Source: CAD feature listing. Evaluate the final solid. Frame: model axes, mm. Face numbers are marked on the shaded views. A direction names the side the tool comes from. Coordinates: 2 decimals unless noted, no trailing zeros. Write each loop counter-clockwise with the first axis right and the second up, starting at its lowest first coordinate (ties: lowest second). Pieces come first, ordered by that corner, then holes. Notation, with made-up numbers: M 57,29.5 L 61,29.5 A27 cw 61,59.5 Z; hole C 21,19 d7. An arc over 180 degrees is marked long. Write item = value, one per line. Start each with the question number.
1. Line query: line 1 along Z through (x, y) = (1.3, 0) (3 decimals); line 2 along Y through (x, z) = (-2, -1.5); line 3 along Y through (x, z) = (3.4, 0) (3 decimals). Output: solid intervals per line, ascending.
2. Section query C-C (x = -2.5). Output: boundary loops of the cut face in (y, z).
3. Section query D-D (z = 3.25). Output: boundary loops of the cut face in (x, y), then the cut area to 3 significant figures.
4. Section query A-A (z = -1.75). Output: boundary loops of the cut face in (x, y).
5. Access query for the marked faces 1, 2 and 3. Directions: +Z, -Z, +X, -X, +Y, -Y. A direction counts if a zero-diameter tool reaches every point of the face in a straight line with its end or side. Return the directions, or none.
6. Section query B-B (y = 1.5). Output: boundary loops of the cut face in (x, z), then the cut area to 3 significant figures.
7. Pull-direction query (X, two-part tool) for the marked faces 4, 5 and 6; classes: pulls with the +X half, pulls with the -X half, needs draft (parallel to the pull), parting line crosses it, or undercut.
8. Pin query (flat end, axial travel): pin 1 Ø2.5 at (y, z) = (0, 0) entering from -X; pin 2 Ø1.1 at (x, y) = (-3.5, 1.5) entering from +Z. Return the tip coordinate at first contact, or that it passes through.
```python
from build123d import *

# Parameters (mm, degrees)
SKETCH052_W          = 12
SKETCH052_H          = 14
PAD011_DEPTH         = 6
POCKET024_DEPTH      = 1
POCKET025_DEPTH      = 5.001
SKETCH055_R          = 2.125
POCKET026_DEPTH      = 6.001
POCKET026_DEPTH_BACK = 6.001
SKETCH056_R          = 4.65
POCKET027_DEPTH      = 1


with BuildPart() as part:
    # Sketch052 → Pad011 (new body, symmetric)
    with BuildSketch(Plane.XY):
        Rectangle(SKETCH052_W, SKETCH052_H)
    extrude(amount=PAD011_DEPTH, both=True)

    # Sketch053 → Pocket024 (cut)
    with BuildSketch(Plane.YZ):
        with BuildLine():
            ThreePointArc((-4.65, 0), (0, -4.65), (4.65, 0))
            Line((4.65, 0), (4.65, 10))
            Line((4.65, 10), (-4.65, 10))
            Line((-4.65, 10), (-4.65, 0))
        make_face()
    extrude(amount=-POCKET024_DEPTH, mode=Mode.SUBTRACT)

    # Sketch054 → Pocket025 (cut, through all)
    with BuildSketch(Plane.YZ.offset(-1)):
        Polygon((0, 4.0414518843), (-3.5, 2.0207259422), (-3.5, -2.0207259422), (0, -4.0414518843), (3.5, -2.0207259422), (3.5, 2.0207259422), align=None)
    extrude(amount=-POCKET025_DEPTH, mode=Mode.SUBTRACT)

    # Sketch055 → Pocket026 (cut, two sides)
    with BuildSketch(Plane.YZ) as pocket026_sk:
        Circle(SKETCH055_R)
    extrude(amount=-POCKET026_DEPTH, mode=Mode.SUBTRACT)
    extrude(pocket026_sk.sketch, amount=POCKET026_DEPTH_BACK, mode=Mode.SUBTRACT)

    # Sketch056 → Pocket027 (cut)
    with BuildSketch(Plane.XY.offset(6)):
        Circle(SKETCH056_R)
    extrude(amount=-POCKET027_DEPTH, mode=Mode.SUBTRACT)


solid = part.part
```
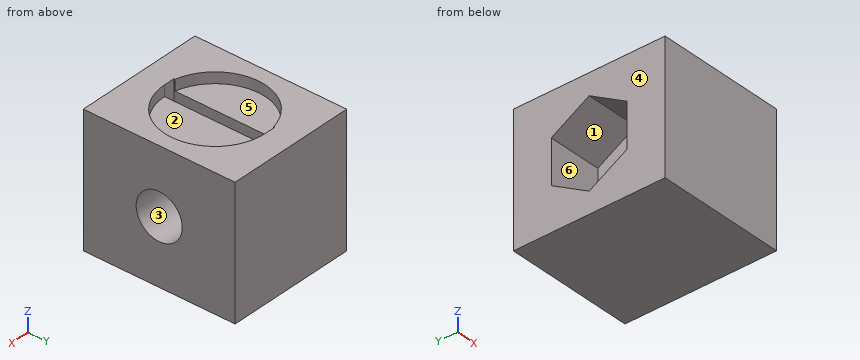
Results are:
q1.line_1 = -6 to -2.125, 2.125 to 5
q1.line_2 = -7 to -3.5, 3.5 to 7
q1.line_3 = -7 to -2.125, 2.125 to 7
q2.outline = M -7,-6 L 7,-6 L 7,6 L 3.92,6 L 3.92,5 L -3.92,5 L -3.92,6 L -7,6 Z; hole M -3.5,-2.02 L 0,-4.04 L 3.5,-2.02 L 3.5,2.02 L 0,4.04 L -3.5,2.02 Z
q3.outline = M -6,-7 L 6,-7 L 6,7 L -6,7 L -6,1.37 L -1,1.37 L -1,4.65 L 0,4.65 L 0,-4.65 L -1,-4.65 L -1,-1.37 L -6,-1.37 Z
q3.area = 145 mm^2
q4.outline = M -6,-7 L 6,-7 L 6,-1.21 L 0,-1.21 L 0,-4.31 L -1,-4.31 L -1,-3.5 L -6,-3.5 Z; M -6,3.5 L -1,3.5 L -1,4.31 L 0,4.31 L 0,1.21 L 6,1.21 L 6,7 L -6,7 Z
q5.face_1 = -X
q5.face_2 = +Z
q5.face_3 = +X, -X
q6.outline = M -6,-6 L 6,-6 L 6,-1.51 L 0,-1.51 L 0,-4.4 L -1,-4.4 L -1,-3.18 L -6,-3.18 Z; M -6,3.18 L -1,3.18 L -1,5 L -4.4,5 L -4.4,6 L -6,6 Z; M 0,1.51 L 6,1.51 L 6,6 L 4.4,6 L 4.4,5 L 0,5 Z
q6.area = 76.0 mm^2
q7.face_4 = pulls with the -X half
q7.face_5 = undercut
q7.face_6 = needs draft
q8.pin_1 = through
q8.pin_2 = 5
